The drawing under review shows one solid part. Ordinate dimensions are in mm from its lowest x, y, z. Round coordinates to 2 decimals unless told otherwise and drop trailing zeros. Order: outer loops, then holes, each group sorted by start corner. A loop starts at its lowest first (then second) coordinate and runs counter-clockwise, first axis right, second up. Notation, with made-up numbers: M 35.5,-8 L 39.5,-8 A34 cw 39.5,23 Z; hole C 78.5,77 d2. An arc over 180 degrees is marked long. Use a Markdown table: item, result.
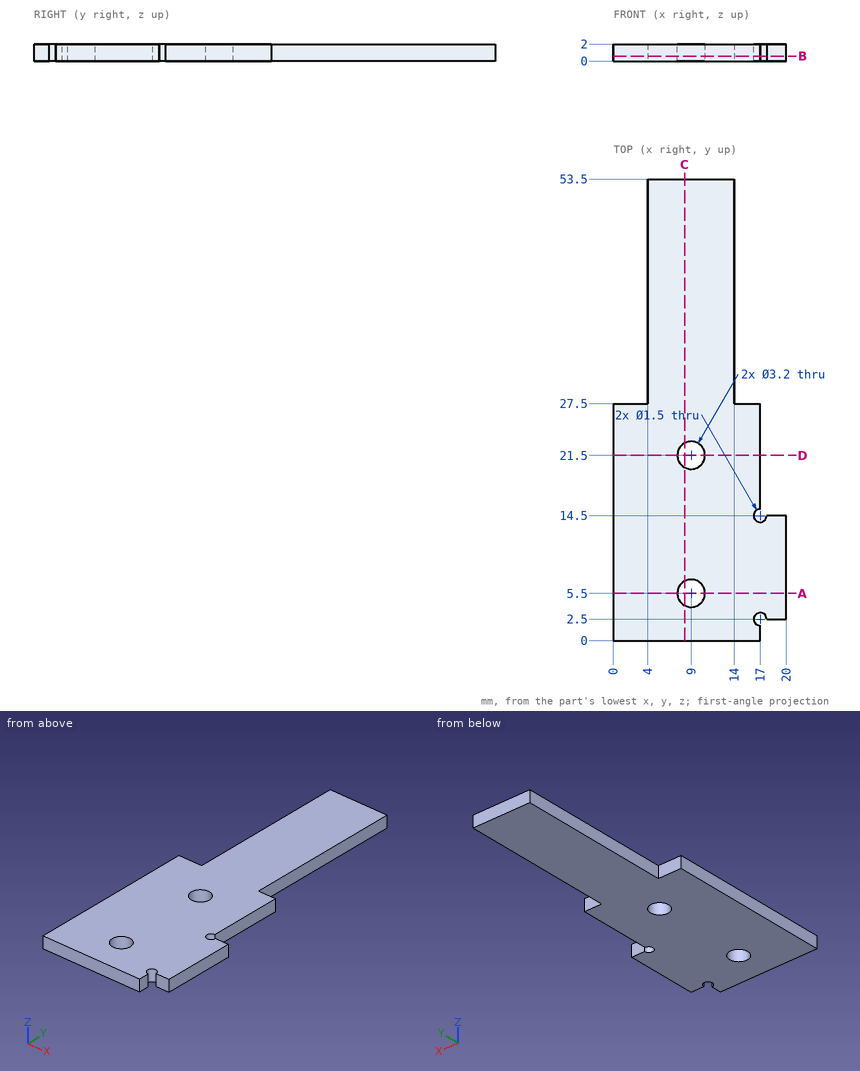
Q1. Clearance check with flat-ended pins moving along their axes: pin 1 (0.6 mm diameter, centred on x = 16, z = 0.5, fed in from +Y); pin 2 (0.6 mm diameter, centred on y = 18.5, z = 1, fed in from +X); pin 3 (0.6 mm diameter, centred on x = 18.5, z = 1, fed in from +Y); pin 4 (1.4 mm diameter, centred on x = 17, y = 14.5, fed in from +Z). State where each tip first meets the part, or that it passes through.
Determined:
| item | result |
|---|---|
| pin 1 | stops at y = 27.5 |
| pin 2 | stops at x = 17 |
| pin 3 | stops at y = 14.5 |
| pin 4 | passes through |
Q2. Add section A-A (y = 5.5). Write out the cut boundary in (x, z), then the cut area to 3 significant figures.
Determined:
| item | result |
|---|---|
| outline | M 0,0 L 7.4,0 L 7.4,2 L 0,2 Z; M 10.6,0 L 20,0 L 20,2 L 10.6,2 Z |
| area | 33.6 mm^2 |
Q3. Wall thickness on line 1 along Y through (x, z) = (9, 0.95); line 2 along X through (y, z) = (34.5, 1.45); line 3 along X through (y, z) = (16, 0.75): over which ranges is each line inside the solid? List them lowest first. Write a range as [from, to].
Determined:
| item | result |
|---|---|
| line 1 | y = [0, 3.9], [7.1, 19.9], [23.1, 53.5] |
| line 2 | x = [4, 14] |
| line 3 | x = [0, 17] |
Q4. Add section B-B (z = 0.6). Write out the cut boundary in (x, y), then the cut area to 3 significant figures.
Determined:
| item | result |
|---|---|
| outline | M 0,0 L 17,0 L 17,1.75 A0.75 cw long 17.75,2.5 L 20,2.5 L 20,14.5 L 17.75,14.5 A0.75 cw long 17,15.25 L 17,27.5 L 14,27.5 L 14,53.5 L 4,53.5 L 4,27.5 L 0,27.5 Z; hole C 9,5.5 d3.2; hole C 9,21.5 d3.2 |
| area | 745 mm^2 |
Q5. Add section D-D (y = 21.5). Write out the cut boundary in (x, z).
Determined:
| item | result |
|---|---|
| outline | M 0,0 L 7.4,0 L 7.4,2 L 0,2 Z; M 10.6,0 L 17,0 L 17,2 L 10.6,2 Z |
Q6. Add section C-C (x = 8.25). Write out the cut boundary in (y, z).
Determined:
| item | result |
|---|---|
| outline | M 0,0 L 4.09,0 L 4.09,2 L 0,2 Z; M 6.91,0 L 20.09,0 L 20.09,2 L 6.91,2 Z; M 22.91,0 L 53.5,0 L 53.5,2 L 22.91,2 Z |
